```python
from build123d import *

# Parameters (mm, degrees)
F0_W      = 80
F0_H      = 100
F1_DEPTH  = 5
F2_W      = 170
F2_H      = 100
F3_DEPTH  = 10
F4_R      = 6
F5_DEPTH  = 10
F7_DEPTH  = 25
F5_FACE_R = 6
F8_DEPTH  = 50


with BuildPart() as f1:
    # F0 (on Front) → F1 (new body, symmetric)
    with BuildSketch(Plane.XZ):
        Rectangle(F0_W, F0_H)
    extrude(amount=F1_DEPTH, both=True)

    # F2 (on face) → F3 (join)
    with BuildSketch(Plane(origin=(0, 0, -50), x_dir=(1, 0, 0), z_dir=(0, 0, -1))):
        with Locations((45, 45)):
            Rectangle(F2_W, F2_H)
    extrude(amount=F3_DEPTH)

    # F4 (on face) → F5 (join)
    with BuildSketch(Plane.XZ.offset(5)):
        with Locations((0, 25)):
            Circle(F4_R)
        with Locations((0, -20)):
            Circle(F4_R)
    extrude(amount=F5_DEPTH)

    # F6 (on face) → F7 (cut)
    with BuildSketch(Plane.XY.offset(-50)):
        with BuildLine():
            ThreePointArc((104, -10), (99.757359, -11.757359), (98, -16))
            Line((98, -16), (98, -76))
            ThreePointArc((98, -76), (99.757359, -80.242641), (104, -82))
            ThreePointArc((104, -82), (108.242641, -80.242641), (110, -76))
            Line((110, -76), (110, -16))
            ThreePointArc((110, -16), (108.242641, -11.757359), (104, -10))
        make_face()
        with BuildLine():
            ThreePointArc((64, -10), (59.757359, -11.757359), (58, -16))
            Line((58, -16), (58, -76))
            ThreePointArc((58, -76), (59.757359, -80.242641), (64, -82))
            ThreePointArc((64, -82), (68.242641, -80.242641), (70, -76))
            Line((70, -76), (70, -16))
            ThreePointArc((70, -16), (68.242641, -11.757359), (64, -10))
        make_face()
    extrude(amount=-F7_DEPTH, mode=Mode.SUBTRACT)

    # F5_face (on face) → F8 (cut)
    with BuildSketch(Plane(origin=(0, -15, 25), x_dir=(1, 0, 0), z_dir=(0, -1, 0))):
        Circle(F5_FACE_R)
        with Locations((0, -45)):
            Circle(F5_FACE_R)
    extrude(amount=-F8_DEPTH, mode=Mode.SUBTRACT)


solid = f1.part
```
Source: CAD feature listing. Evaluate the final solid. Frame: model axes, mm. A direction names the side the tool comes from. Round coordinates to 2 decimals unless told otherwise and drop trailing zeros. Loops run counter-clockwise (first coordinate to the right, second up) from the corner with the lowest first, then second, coordinate; pieces in that order, holes last.
(1) Section query B-B (z = -20). Output: boundary loops of the cut face in (x, y).
From the geometry:
outline: (-40, -5) - (-6, -5) - (-6, 5) - (-40, 5) - close; (6, -5) - (40, -5) - (40, 5) - (6, 5) - close
(2) Section query D-D (x = -24.5). Output: boundary loops of the cut face in (y, z), and give its area (3 significant figures).
From the geometry:
outline: (-95, -60) - (5, -60) - (5, 50) - (-5, 50) - (-5, -50) - (-95, -50) - close
area: 2,000 mm2
(3) Pull-direction query (X, two-part tool) for faces 5 (the cylindrical face through (-1.301, -0.07, 19.143)), 6 (the flat face through (44, -95, -55)), 7 (the flat face through (-40, -4, -21)); classes: +X half, -X half, draft (parallel to the pull), parting line (faces both ways), or undercut.
From the geometry:
face 5: undercut
face 6: draft
face 7: -X half
(4) Contact query for flat-ended pins moving along their axis: pin 1 Ø4 at (x, y) = (28.5, -48) entering from +Z; pin 2 Ø19 at (x, z) = (0, -20) entering from -Y; pin 3 Ø3 at (y, z) = (0, 0) entering from +X. Output: stop coordinate, or through.
From the geometry:
pin 1: stops at z = -50
pin 2: stops at y = -5
pin 3: stops at x = 40
(5) Access query for faces 1 (the flat face through (40, 0, -1)), 2 (the flat face through (58, -46, -55)), 3 (the flat face through (-1, -5, 1)), 4 (the flat face through (-1, 0, 50)). Directions: +Z, -Z, +X, -X, +Y, -Y. A direction counts if a zero-diameter tool reaches every point of the face in a straight line with its end or side. Return the directions, or none.
From the geometry:
face 1: +Z, +X, +Y, -Y
face 2: +Z, -Z
face 3: +Z, +X, -X, -Y
face 4: +Z, +X, -X, +Y, -Y
(6) Material intervals for probe 1 along Z at (x, y) = (0, -0.25); probe 2 along Z at (x, y) = (119, -26.5); probe 3 along Y at (x, z) = (33.5, -2.5), sorted ascending.
From the geometry:
probe 1: z = -60 to -26, -14 to 19, 31 to 50
probe 2: z = -60 to -50
probe 3: y = -5 to 5
(7) Section query A-A (y = -51.5). Output: boundary loops of the cut face in (x, z).
From the geometry:
outline: (-40, -60) - (58, -60) - (58, -50) - (-40, -50) - close; (70, -60) - (98, -60) - (98, -50) - (70, -50) - close; (110, -60) - (130, -60) - (130, -50) - (110, -50) - close
(8) Section query C-C (x = 0). Output: boundary loops of the cut face in (y, z), and give its area (3 significant figures).
From the geometry:
outline: (-95, -60) - (5, -60) - (5, -26) - (-5, -26) - (-5, -50) - (-95, -50) - close; (-5, -14) - (5, -14) - (5, 19) - (-5, 19) - close; (-5, 31) - (5, 31) - (5, 50) - (-5, 50) - close
area: 1,760 mm2
